Build history of the part. All positions in model axes, mm. Face numbers are marked on the shaded views. Give positions to 0.01 mm unless a question says otherwise; leave off trailing zeros. Order: outer loops, then holes, each group sorted by start corner. A loop starts at its lowest first (then second) coordinate and runs counter-clockwise, first axis right, second up. Notation, with made-up numbers: (79.5, 86.25) - (105.5, 86.25) arc R38 cw to (105.5, 125.25) - close; hole circle Ø8 at (48, -35.75). An arc over 180 degrees is marked (long way). Use a Markdown table: item, result.
from build123d import *

# Parameters (mm, degrees)
BOSS_EXTRUDE1_DEPTH = 2.5
CUT_EXTRUDE2_REACH  = 21.385
SKETCH2_R           = 2.2
CHAMFER1_SIZE       = 2
FILLET1_R           = 2.5


with BuildPart() as part:
    # Sketch1 → Boss-Extrude1 (new body)
    with BuildSketch(Plane(origin=(0, 0, 0), x_dir=(1, 0, 0), z_dir=(0, 1, 0))):
        Polygon((-17.7, -5), (-5, -7.5), (5, -7.5), (17.7, -5), (17.7, 5), (5, 7.5), (-5, 7.5), (-17.7, 5), align=None)
    extrude(amount=BOSS_EXTRUDE1_DEPTH)

    # Sketch2 → Cut-Extrude2 (cut, up to next)
    with BuildSketch(Plane(origin=(0, 2.5, 0), x_dir=(1, 0, 0), z_dir=(0, 1, 0)), mode=Mode.PRIVATE) as cut_extrude2_sk1:
        with Locations(Location((-12.7, 0, 0), (0, 0, 270))):
            Circle(SKETCH2_R)
    cut_extrude2_tool1 = extrude(cut_extrude2_sk1.sketch, amount=-CUT_EXTRUDE2_REACH, mode=Mode.PRIVATE) & part.part
    # Sketch2 → Cut-Extrude2 (cut, up to next)
    with BuildSketch(Plane(origin=(0, 2.5, 0), x_dir=(1, 0, 0), z_dir=(0, 1, 0)), mode=Mode.PRIVATE) as cut_extrude2_sk2:
        with Locations(Location((12.7, 0, 0), (0, 0, 270))):
            Circle(SKETCH2_R)
    cut_extrude2_tool2 = extrude(cut_extrude2_sk2.sketch, amount=-CUT_EXTRUDE2_REACH, mode=Mode.PRIVATE) & part.part
    add(cut_extrude2_tool1.solids().sort_by_distance((-12.7, 2.5, 0))[0], mode=Mode.SUBTRACT)
    add(cut_extrude2_tool2.solids().sort_by_distance((12.7, 2.5, 0))[0], mode=Mode.SUBTRACT)

    # Chamfer1
    chamfer1_edges = [part.edges().sort_by_distance(p)[0] for p in [
        (-12.7, 2.5, -2.2),
        (12.7, 2.5, -2.2),
    ]]
    chamfer(chamfer1_edges, length=CHAMFER1_SIZE)

    # Fillet1
    fillet1_edges = [part.edges().sort_by_distance(p)[0] for p in [
        (5, 1.25, -7.5),
        (17.7, 1.25, -5),
        (17.7, 1.25, 5),
        (5, 1.25, 7.5),
        (-5, 1.25, 7.5),
        (-17.7, 1.25, 5),
        (-17.7, 1.25, -5),
        (-5, 1.25, -7.5),
    ]]
    fillet(fillet1_edges, radius=FILLET1_R)


solid = part.part
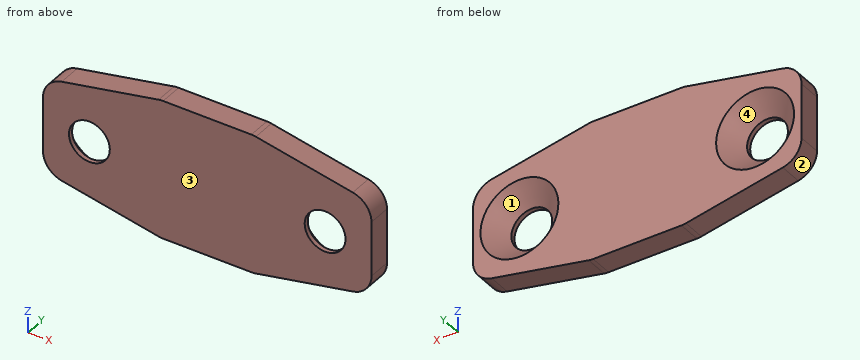
1) Slice it at A-A (y = 1). Write the cut outline in (x, z), and give its area (3 significant figures).
Computed:
| item | result |
|---|---|
| outline | (-17.7, -2.94) arc R2.5 ccw to (-15.68, -5.4) - (-5.24, -7.45) arc R2.5 ccw to (-4.76, -7.5) - (4.76, -7.5) arc R2.5 ccw to (5.24, -7.45) - (15.68, -5.4) arc R2.5 ccw to (17.7, -2.94) - (17.7, 2.94) arc R2.5 ccw to (15.68, 5.4) - (5.24, 7.45) arc R2.5 ccw to (4.76, 7.5) - (-4.76, 7.5) arc R2.5 ccw to (-5.24, 7.45) - (-15.68, 5.4) arc R2.5 ccw to (-17.7, 2.94) - close; hole circle Ø5.4 at (-12.7, 0); hole circle Ø5.4 at (12.7, 0) |
| area | 418 mm² |
2) Slice it at B-B (z = 0). Write the cut outline in (x, y).
Computed:
| item | result |
|---|---|
| outline | (-17.7, 0) - (-14.9, 0) - (-14.9, 0.5) - (-16.9, 2.5) - (-17.7, 2.5) - close; (-10.5, 0) - (10.5, 0) - (10.5, 0.5) - (8.5, 2.5) - (-8.5, 2.5) - (-10.5, 0.5) - close; (14.9, 0) - (17.7, 0) - (17.7, 2.5) - (16.9, 2.5) - (14.9, 0.5) - close |
3) Pin check, flat tip, straight feed: P1, Ø3.5, axis at x = 12.7, z = 0, coming from the -Y side. Stop position of the tip, or through.
Computed:
| item | result |
|---|---|
| P1 | passes through |
4) Two-plate mould, pull along X, no slides. Class the marked faces 1, 2, 3 and 4: +X half, -X half, draft (parallel to the pull), parting line (faces both ways), or undercut.
Computed:
| item | result |
|---|---|
| face 1 | undercut |
| face 2 | -X half |
| face 3 | draft |
| face 4 | undercut |
5) Wall check: line 1 (X direction, y = 0.4, z = 0); line 2 (X direction, y = 1.6, z = 0.5); line 3 (Z direction, x = -15, y = 1.25). Give the ranges that are in metal, low to high. Write a range as from..to.
Computed:
| item | result |
|---|---|
| line 1 | x = -17.7..-14.9, -10.5..10.5, 14.9..17.7 |
| line 2 | x = -17.7..-15.96, -9.44..9.44, 15.96..17.7 |
| line 3 | z = -5.53..-1.85, 1.85..5.53 |
6) Slice it at C-C (x = -12.7). Write the cut outline in (y, z), and give its area (3 significant figures).
Computed:
| item | result |
|---|---|
| outline | (0, -5.98) - (2.5, -5.98) - (2.5, -4.2) - (0.5, -2.2) - (0, -2.2) - close; (0, 2.2) - (0.5, 2.2) - (2.5, 4.2) - (2.5, 5.98) - (0, 5.98) - close |
| area | 14.9 mm² |
7) Slice it at D-D (z = 6). Write the cut outline in (x, y), and give its area (3 significant figures).
Computed:
| item | result |
|---|---|
| outline | (-12.62, 0) - (12.62, 0) - (12.62, 2.5) - (-12.62, 2.5) - close |
| area | 63.1 mm² |
